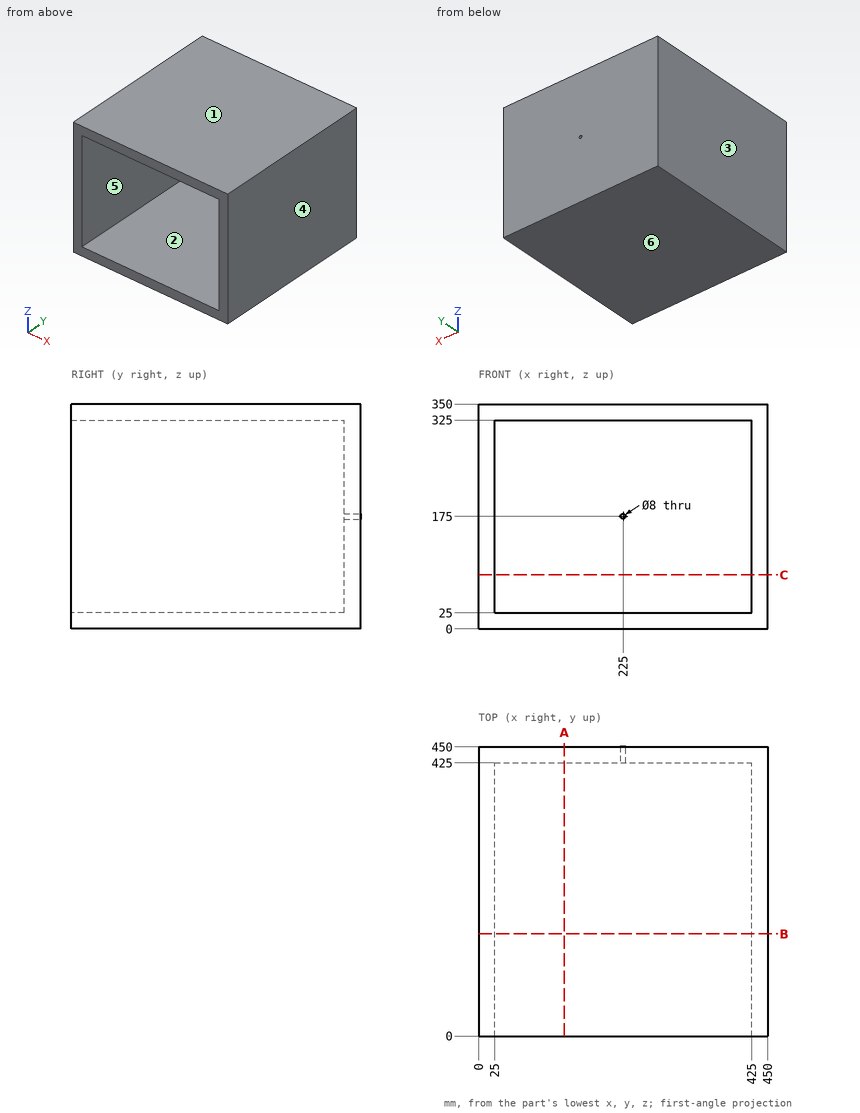
Job drawing, mm, ordinate dimensions from the low corner. One solid piece. A direction names the side the tool comes from. Coordinates: 2 decimals unless noted, no trailing zeros. Write each loop counter-clockwise with the first axis right and the second up, starting at its lowest first coordinate (ties: lowest second). Pieces come first, ordered by that corner, then holes. Notation, with made-up numbers: (0.25, -12) - (46.25, -12) arc R18 ccw to (46.25, -2) - close; hole circle Ø1 at (65, -33.75). An arc over 180 degrees is marked (long way). Use a Markdown table: item, result. Add a question column.
Item 1: Band-saw the part on B-B, the plane y = 159. Give the cut face in (x, z).
Item 2: Band-saw the part on A-A, the plane x = 133.5. Give the cut face in (y, z).
Item 3: Band-saw the part on C-C, the plane z = 84. Give the cut face in (x, y), and give its area (3 significant figures).
Item 4: Drill centre lines: L1, parallel to Z at x = 79, y = 331; L2, parallel to X at y = 283, z = 149; L3, parallel to Z at x = 225, y = 430. Where is each one in solid material? Low to high. Write a range as from..to.
Item 5: 3-axis set-ups, long thin cutter, end or side, ignore diameter. For the marked faces 1 and 2: which of +Z, -Z, +X, -X, +Y, -Y reach the whole face in a straight line?
Item 6: Mould opens along X. For the marked faces 3, 4, 5 and 6 say: pulls with the +X half, pulls with the -X half, needs draft (parallel to the pull), parting line crosses it, or undercut.
Item 7: Flat gauge pin, fed straight in: pin 1 (1.5 mm diameter, centred on x = 305, z = 80.5, fed in from -Y). Where does the tip first touch, or does it go through?
Numbers:
| question | item | result |
|---|---|---|
| 1 | outline | (0, 0) - (450, 0) - (450, 350) - (0, 350) - close; hole (25, 25) - (425, 25) - (425, 325) - (25, 325) - close |
| 2 | outline | (0, 0) - (450, 0) - (450, 350) - (0, 350) - (0, 325) - (425, 325) - (425, 25) - (0, 25) - close |
| 3 | outline | (0, 0) - (25, 0) - (25, 425) - (425, 425) - (425, 0) - (450, 0) - (450, 450) - (0, 450) - close |
| 3 | area | 32,500 mm2 |
| 4 | L1 | 0..25, 325..350 |
| 4 | L2 | 0..25, 425..450 |
| 4 | L3 | 0..171, 179..350 |
| 5 | face 1 | +Z, +X, -X, +Y, -Y |
| 5 | face 2 | -Y |
| 6 | face 3 | pulls with the -X half |
| 6 | face 4 | pulls with the +X half |
| 6 | face 5 | undercut |
| 6 | face 6 | needs draft |
| 7 | pin 1 | y = 425 |
